```python
from build123d import *

# Parameters (mm, degrees)
SKETCH_1_R      = 1.6
EXTRUDE_1_DEPTH = 3
SKETCH_6_W      = 13
SKETCH_6_H      = 4
SKETCH_6_R      = 1
EXTRUDE_3_DEPTH = 3
FILLET_1_R      = 3


with BuildPart() as part:
    # ｽｹｯﾁ1 → ﾎﾞｽ - 押し出し1 (new body)
    with BuildSketch(Plane.XY):
        with BuildLine():
            Line((-26, 0), (26, 0))
            ThreePointArc((26, 0), (31, -5), (36, 0))
            Line((36, 0), (36, 7))
            Line((36, 7), (-36, 7))
            Line((-36, 7), (-36, 0))
            ThreePointArc((-36, 0), (-31, -5), (-26, 0))
        make_face()
        with Locations((-31, 0)):
            Circle(SKETCH_1_R, mode=Mode.SUBTRACT)
        with Locations((31, 0)):
            Circle(SKETCH_1_R, mode=Mode.SUBTRACT)
    extrude(amount=EXTRUDE_1_DEPTH)

    # ｽｹｯﾁ6 → ﾎﾞｽ - 押し出し3 (add)
    with BuildSketch(Plane(origin=(0, 7, 0), x_dir=(1, 0, 0), z_dir=(0, 1, 0))):
        with Locations((0, 2)):
            Rectangle(SKETCH_6_W, SKETCH_6_H)
        with Locations(Location((-3.25, 2, 0), (0, 0, 180))):
            Circle(SKETCH_6_R, mode=Mode.SUBTRACT)
        with Locations(Location((3.25, 2, 0), (0, 0, 180))):
            Circle(SKETCH_6_R, mode=Mode.SUBTRACT)
    extrude(amount=-EXTRUDE_3_DEPTH)

    # ﾌｨﾚｯﾄ1
    fillet_1_edges = [part.edges().sort_by_distance(p)[0] for p in [
        (-36, 7, 1.5),
        (36, 7, 1.5),
    ]]
    fillet(fillet_1_edges, radius=FILLET_1_R)


solid = part.part
```
The model under review builds one solid part; all positions refer to its coordinate system, in mm. A direction names the side the tool comes from. Round coordinates to 2 decimals unless told otherwise and drop trailing zeros. Order: outer loops, then holes, each group sorted by start corner. A loop starts at its lowest first (then second) coordinate and runs counter-clockwise, first axis right, second up. Notation, with made-up numbers: (-27.5, 13) - (7.5, 13) arc R25 cw to (7.5, 39) - close; hole circle Ø5 at (50, 56.5). An arc over 180 degrees is marked (long way). Answer in a Markdown table with one row per item.
(1) Machinability: for faces 1 (the face through (6.5, 6, -2)), 2 (the face through (0, 0, 1)), 3 (the face through (0, 4, -2)), 4 (the face through (-6.5, 6, -2)), which of the approach directions +Z, -Z, +X, -X, +Y, -Y give a long, thin tool a straight path to every point of the face, cutting with its end or side? Answer none if there is none.
Result set:
| item | result |
|---|---|
| face 1 | -Z, +X, +Y, -Y |
| face 2 | +Z, -Z, -Y |
| face 3 | -Z, +X, -X, -Y |
| face 4 | -Z, -X, +Y, -Y |
(2) Take a section at B-B on z = -2. Write out the cut boundary in (x, y).
Result set:
| item | result |
|---|---|
| outline | (-6.5, 4) - (-4.25, 4) - (-4.25, 7) - (-6.5, 7) - close; (-2.25, 4) - (2.25, 4) - (2.25, 7) - (-2.25, 7) - close; (4.25, 4) - (6.5, 4) - (6.5, 7) - (4.25, 7) - close |
(3) Clearance check with flat-ended pins moving along their axes: P1, Ø1.5, axis at y = -3, z = 0.5, coming from the -X side; P2, Ø2.5, axis at x = 8.5, z = 1.5, coming from the -Y side; P3, Ø2.5, axis at x = 3.25, z = -2, coming from the -Y side; P4, Ø1.8, axis at x = -3.25, z = -2, coming from the -Y side. State where each tip first meets the part, or that it passes through.
Result set:
| item | result |
|---|---|
| P1 | stops at x = -35.47 |
| P2 | stops at y = 0 |
| P3 | stops at y = 4 |
| P4 | passes through |
(4) For line 1 (Y direction, x = 31, z = 1.8); line 2 (Z direction, x = 3.25, y = 6); line 3 (Y direction, x = -3, z = -3.25), list the stretches that pass through material, from the lowest coordinate up. Write a range as from..to.
Result set:
| item | result |
|---|---|
| line 1 | y = -5..-1.6, 1.6..7 |
| line 2 | z = -4..-3, -1..3 |
| line 3 | y = 4..7 |
(5) Mouldability with a two-part tool opening along Y and no side actions: class faces 5 (the face through (-32.6, 0.07, 1.48)), 6 (the face through (-35.14, 6.1, 1.52)), 7 (the face through (-31, -5, 1)) as released by +Y, released by -Y, zero draft, split by the parting line, or undercut.
Result set:
| item | result |
|---|---|
| face 5 | undercut |
| face 6 | released by +Y |
| face 7 | released by -Y |
(6) Take a section at A-A on x = -31. Write out the cut boundary in (y, z), plus the area to 3 significant figures.
Result set:
| item | result |
|---|---|
| outline | (-5, 0) - (-1.6, 0) - (-1.6, 3) - (-5, 3) - close; (1.6, 0) - (7, 0) - (7, 3) - (1.6, 3) - close |
| area | 26.4 mm2 |
(7) Take a section at D-D on y = 5.75. Write out the cut boundary in (x, z), plus the area to 3 significant figures.
Result set:
| item | result |
|---|---|
| outline | (-35.44, 0) - (-6.5, 0) - (-6.5, -4) - (6.5, -4) - (6.5, 0) - (35.44, 0) - (35.44, 3) - (-35.44, 3) - close; hole circle Ø2 at (-3.25, -2); hole circle Ø2 at (3.25, -2) |
| area | 258 mm2 |
(8) Take a section at C-C on y = -3.25. Write out the cut boundary in (x, z).
Result set:
| item | result |
|---|---|
| outline | (-34.8, 0) - (-27.2, 0) - (-27.2, 3) - (-34.8, 3) - close; (27.2, 0) - (34.8, 0) - (34.8, 3) - (27.2, 3) - close |
